```python
from build123d import *

# Parameters (mm, degrees)
SKETCH7_R           = 1.5
BOSS_EXTRUDE1_DEPTH = 3.5
SKETCH10_W          = 18
SKETCH10_H          = 10
SKETCH10_R          = 1.25
BOSS_EXTRUDE3_DEPTH = 3.5


with BuildPart() as part:
    # Sketch7 → Boss-Extrude1 (new body)
    with BuildSketch(Plane.XY):
        with BuildLine():
            Line((-4, 60), (-4, 70))
            Line((-4, 70), (-44.142135624, 70))
            Line((-44.142135624, 70), (-57.5, 83.35))
            Line((-57.5, 83.35), (-57.5, 93.35))
            Line((-57.5, 93.35), (57.5, 93.35))
            Line((57.5, 93.35), (57.5, 83.35))
            Line((57.5, 83.35), (44.142135624, 70))
            Line((44.142135624, 70), (4, 70))
            Line((4, 70), (4, 60))
            ThreePointArc((4, 60), (0, 56), (-4, 60))
        make_face()
        with Locations((0, 60)):
            Circle(SKETCH7_R, mode=Mode.SUBTRACT)
        with BuildLine():
            Line((22.5, 89.35), (-22.5, 89.35))
            ThreePointArc((-22.5, 89.35), (-27, 84.85), (-22.5, 80.35))
            Line((-22.5, 80.35), (22.5, 80.35))
            ThreePointArc((22.5, 80.35), (27, 84.85), (22.5, 89.35))
        make_face(mode=Mode.SUBTRACT)
    extrude(amount=BOSS_EXTRUDE1_DEPTH)

    # Sketch10 → Boss-Extrude3 (add)
    with BuildSketch(Plane(origin=(0, 93.35, 0), x_dir=(1, 0, 0), z_dir=(0, 1, 0))):
        with Locations((-48.5, 5)):
            Rectangle(SKETCH10_W, SKETCH10_H)
        with Locations((-53.5, 5)):
            Circle(SKETCH10_R, mode=Mode.SUBTRACT)
        with Locations((-43.5, 5)):
            Circle(SKETCH10_R, mode=Mode.SUBTRACT)
        with Locations((48.5, 5)):
            Rectangle(SKETCH10_W, SKETCH10_H)
        with Locations((43.5, 5)):
            Circle(SKETCH10_R, mode=Mode.SUBTRACT)
        with Locations((53.5, 5)):
            Circle(SKETCH10_R, mode=Mode.SUBTRACT)
    extrude(amount=-BOSS_EXTRUDE3_DEPTH)


solid = part.part
```
Check sheet for the modelled part. Datum: model origin and axes. Units: mm. A direction names the side the tool comes from. Round coordinates to 2 decimals unless told otherwise and drop trailing zeros. Loops run counter-clockwise (first coordinate to the right, second up) from the corner with the lowest first, then second, coordinate; pieces in that order, holes last. Notation, with made-up numbers: (50, -19.75) - (108, -19.75) arc R26 cw to (108, 18.25) - close; hole circle Ø5 at (34.25, 15.5). An arc over 180 degrees is marked (long way). Write item = value, one per line. Start each with the question number.
Q1. Section check C-C (x = -53.5). Record the boundary of the cut face in (y, z), plus the area to 3 significant figures.
Q2. Section check D-D (y = 75.5). Record the boundary of the cut face in (x, z).
Q3. Depth check by flat-ended pin: P1, Ø10, axis at x = -32, y = 74, coming from the -Z side; P2, Ø4, axis at x = 18.5, y = 80.5, coming from the +Z side; P3, Ø2, axis at x = -53.5, z = -5, coming from the -Y side; P4, Ø1.5, axis at x = -23, z = 1, coming from the -Y side. Enter the tip coordinate at first touch or a pass-through.
Q4. Section check A-A (z = -7.5). Record the boundary of the cut face in (x, y), plus the area to 3 significant figures.
Q5. Section check B-B (y = 84.85). Record the boundary of the cut face in (x, z), plus the area to 4 significant figures.
Q6. Thickness scan on L1, parallel to Y at x = 0, z = 2.2; L2, parallel to X at y = 91.6, z = -5; L3, parallel to Y at x = -16, z = 0.5. Record the ranges inside material, lowest first.
Q7. Release check for a two-part mould opening along X. For faces 1 (the face through (-49, 89.85, -5)), 2 (the face through (-52.31, 91.62, -5.38)), 3 (the face through (0, 56, 2)), 4 (the face through (-57.5, 91, -2)) record: pulls with the +X half, pulls with the -X half, needs draft (parallel to the pull), parting line crosses it, or undercut.
Q8. Access from +Z, -Z, +X, -X, +Y, -Y to the whole of each face (thin tool, end or side, straight path). Record for faces 5 (the face through (57.5, 91, -2)), 6 (the face through (-27, 84.9, 1.7)), 7 (the face through (1, 79, 0)), 8 (the face through (-39.5, 92, -5)), 9 (the face through (-24, 70, 2)).
Derived:
q1.outline = (79.35, 0) - (89.85, 0) - (89.85, -3.75) - (93.35, -3.75) - (93.35, 3.5) - (79.35, 3.5) - close; (89.85, -10) - (93.35, -10) - (93.35, -6.25) - (89.85, -6.25) - close
q1.area = 75.2 mm^2
q2.outline = (-49.65, 0) - (49.65, 0) - (49.65, 3.5) - (-49.65, 3.5) - close
q3.P1 = 0
q3.P2 = 3.5
q3.P3 = through
q3.P4 = 70
q4.outline = (-57.5, 89.85) - (-39.5, 89.85) - (-39.5, 93.35) - (-57.5, 93.35) - close; (39.5, 89.85) - (57.5, 89.85) - (57.5, 93.35) - (39.5, 93.35) - close
q4.area = 126 mm^2
q5.outline = (-57.5, 0) - (-27, 0) - (-27, 3.5) - (-57.5, 3.5) - close; (27, 0) - (57.5, 0) - (57.5, 3.5) - (27, 3.5) - close
q5.area = 213.5 mm^2
q6.L1 = 56 to 58.5, 61.5 to 80.35, 89.35 to 93.35
q6.L2 = -57.5 to -54.75, -52.25 to -44.75, -42.25 to -39.5, 39.5 to 42.25, 44.75 to 52.25, 54.75 to 57.5
q6.L3 = 70 to 80.35, 89.35 to 93.35
q7.face_1 = needs draft
q7.face_2 = undercut
q7.face_3 = parting line crosses it
q7.face_4 = pulls with the -X half
q8.face_5 = +Z, -Z, +X, +Y, -Y
q8.face_6 = +Z, -Z
q8.face_7 = -Z, -Y
q8.face_8 = -Z, +Y, -Y
q8.face_9 = +Z, -Z, -X, -Y
